from build123d import *

# Parameters (mm, degrees)
SKETCH_W        = 200
SKETCH_H        = 200
SKETCH_W_2      = 180
SKETCH_H_2      = 180
PAD_DEPTH       = 50
SKETCH001_W     = 40
SKETCH001_H     = 40
POCKET_DEPTH    = 2
SKETCH002_R     = 20
POCKET001_DEPTH = 8
SKETCH003_W     = 22
SKETCH003_H     = 12
POCKET002_DEPTH = 10
SKETCH004_R     = 5
POCKET003_DEPTH = 10
SKETCH005_W     = 15
SKETCH005_H     = 15
POCKET004_DEPTH = 2
SKETCH006_R     = 0.75
POCKET005_DEPTH = 10
POCKET006_DEPTH = 10
SKETCH008_W     = 10
SKETCH008_H     = 10
SKETCH008_R     = 1.8
PAD001_DEPTH    = 10
FILLET_R        = 1
SKETCH009_R     = 1.2
POCKET007_DEPTH = 5
SKETCH010_W     = 110
SKETCH010_H     = 40
POCKET008_DEPTH = 5
SKETCH011_W     = 110
SKETCH011_H     = 40
POCKET009_DEPTH = 5
SKETCH012_W     = 110
SKETCH012_H     = 40
POCKET010_DEPTH = 5


with BuildPart() as part:
    # Sketch → Pad (new body)
    with BuildSketch(Plane.XY):
        with Locations((100, 100)):
            Rectangle(SKETCH_W, SKETCH_H)
        with Locations((100, 100)):
            Rectangle(SKETCH_W_2, SKETCH_H_2, mode=Mode.SUBTRACT)
    extrude(amount=PAD_DEPTH)

    # Sketch001 (on Face1 of Pad) → Pocket (cut)
    with BuildSketch(Plane.XZ):
        with Locations((160, 25)):
            Rectangle(SKETCH001_W, SKETCH001_H)
    extrude(amount=-POCKET_DEPTH, mode=Mode.SUBTRACT)

    # Sketch002 (on Face15 of Pocket) → Pocket001 (cut)
    with BuildSketch(Plane.XZ.offset(-2)):
        with Locations((160, 25)):
            Circle(SKETCH002_R)
    extrude(amount=-POCKET001_DEPTH, mode=Mode.SUBTRACT)

    # Sketch003 (on Face1 of Pocket001) → Pocket002 (cut)
    with BuildSketch(Plane.XZ):
        with Locations((119, 11)):
            Rectangle(SKETCH003_W, SKETCH003_H)
    extrude(amount=-POCKET002_DEPTH, mode=Mode.SUBTRACT)

    # Sketch004 (on Face1 of Pocket002) → Pocket003 (cut)
    with BuildSketch(Plane.XZ):
        with Locations((93, 11)):
            Circle(SKETCH004_R)
    extrude(amount=-POCKET003_DEPTH, mode=Mode.SUBTRACT)

    # Sketch005 (on Face16 of Pocket003) → Pocket004 (cut)
    with BuildSketch(Plane(origin=(0, 10, 0), x_dir=(-1, 0, 0), z_dir=(0, 1, 0))):
        with Locations((-93, 11)):
            Rectangle(SKETCH005_W, SKETCH005_H)
    extrude(amount=-POCKET004_DEPTH, mode=Mode.SUBTRACT)

    # Sketch006 (on Face4 of Pocket004) → Pocket005 (cut)
    with BuildSketch(Plane.XY.offset(50)):
        with Locations((5, 5)):
            Circle(SKETCH006_R)
        with Locations((195, 5)):
            Circle(SKETCH006_R)
        with Locations((195, 195)):
            Circle(SKETCH006_R)
        with Locations((5, 195)):
            Circle(SKETCH006_R)
    extrude(amount=-POCKET005_DEPTH, mode=Mode.SUBTRACT)

    # Sketch007 (on Face15 of Pocket005) → Pocket006 (cut)
    with BuildSketch(Plane(origin=(0, 200, 0), x_dir=(-1, 0, 0), z_dir=(0, 1, 0))):
        with BuildLine():
            ThreePointArc((-38, 10), (-36.5, 8.5), (-35, 10))
            Line((-35, 10), (-35, 40))
            ThreePointArc((-35, 40), (-36.5, 41.5), (-38, 40))
            Line((-38, 10), (-38, 40))
        make_face()
        with BuildLine():
            ThreePointArc((-33, 10), (-31.5, 8.5), (-30, 10))
            Line((-30, 10), (-30, 40))
            ThreePointArc((-30, 40), (-31.5, 41.5), (-33, 40))
            Line((-33, 10), (-33, 40))
        make_face()
        with BuildLine():
            ThreePointArc((-28, 10), (-26.5, 8.5), (-25, 10))
            Line((-25, 10), (-25, 40))
            ThreePointArc((-25, 40), (-26.5, 41.5), (-28, 40))
            Line((-28, 10), (-28, 40))
        make_face()
        with BuildLine():
            ThreePointArc((-165, 10), (-163.5, 8.5), (-162, 10))
            Line((-162, 10), (-162, 40))
            ThreePointArc((-162, 40), (-163.5, 41.5), (-165, 40))
            Line((-165, 10), (-165, 40))
        make_face()
        with BuildLine():
            ThreePointArc((-170, 10), (-168.5, 8.5), (-167, 10))
            Line((-167, 10), (-167, 40))
            ThreePointArc((-167, 40), (-168.5, 41.5), (-170, 40))
            Line((-170, 10), (-170, 40))
        make_face()
        with BuildLine():
            ThreePointArc((-175, 10), (-173.5, 8.5), (-172, 10))
            Line((-172, 10), (-172, 40))
            ThreePointArc((-172, 40), (-173.5, 41.5), (-175, 40))
            Line((-175, 10), (-175, 40))
        make_face()
    extrude(amount=-POCKET006_DEPTH, mode=Mode.SUBTRACT)

    # Sketch008 (on Face3 of Pocket006) → Pad001 (join)
    with BuildSketch(Plane(origin=(0, 0, 0), x_dir=(1, 0, 0), z_dir=(0, 0, -1))):
        with Locations((185, -15)):
            Rectangle(SKETCH008_W, SKETCH008_H)
        with Locations((185, -15)):
            Circle(SKETCH008_R, mode=Mode.SUBTRACT)
        with Locations((185, -185)):
            Rectangle(SKETCH008_W, SKETCH008_H)
        with Locations((185, -185)):
            Circle(SKETCH008_R, mode=Mode.SUBTRACT)
        with Locations((15, -15)):
            Rectangle(SKETCH008_W, SKETCH008_H)
        with Locations((15, -15)):
            Circle(SKETCH008_R, mode=Mode.SUBTRACT)
        with Locations((15, -185)):
            Rectangle(SKETCH008_W, SKETCH008_H)
        with Locations((15, -185)):
            Circle(SKETCH008_R, mode=Mode.SUBTRACT)
    extrude(amount=-PAD001_DEPTH)

    # Fillet
    fillet_edges = [part.edges().sort_by_distance(p)[0] for p in [
        (180, 20, 5),
        (20, 20, 5),
        (180, 180, 5),
        (20, 180, 5),
    ]]
    fillet(fillet_edges, radius=FILLET_R)

    # Sketch009 (on Face8 of Fillet) → Pocket007 (cut)
    with BuildSketch(Plane(origin=(0, 10, 0), x_dir=(-1, 0, 0), z_dir=(0, 1, 0))):
        with Locations((-144, 9)):
            Circle(SKETCH009_R)
        with Locations((-176, 41)):
            Circle(SKETCH009_R)
        with Locations((-176, 9)):
            Circle(SKETCH009_R)
        with Locations((-144, 41)):
            Circle(SKETCH009_R)
    extrude(amount=-POCKET007_DEPTH, mode=Mode.SUBTRACT)

    # Sketch010 (on Face22 of Pocket007) → Pocket008 (cut)
    with BuildSketch(Plane.YZ.offset(200)):
        with Locations((100, 25)):
            Rectangle(SKETCH010_W, SKETCH010_H)
    extrude(amount=-POCKET008_DEPTH, mode=Mode.SUBTRACT)

    # Sketch011 (on Face20 of Pocket008) → Pocket009 (cut)
    with BuildSketch(Plane(origin=(0, 0, 0), x_dir=(0, -1, 0), z_dir=(-1, 0, 0))):
        with Locations((-100, 25)):
            Rectangle(SKETCH011_W, SKETCH011_H)
    extrude(amount=-POCKET009_DEPTH, mode=Mode.SUBTRACT)

    # Sketch012 (on Face21 of Pocket009) → Pocket010 (cut)
    with BuildSketch(Plane(origin=(0, 200, 0), x_dir=(-1, 0, 0), z_dir=(0, 1, 0))):
        with Locations((-100, 25)):
            Rectangle(SKETCH012_W, SKETCH012_H)
    extrude(amount=-POCKET010_DEPTH, mode=Mode.SUBTRACT)


solid = part.part
Work out the finished part from the listing and answer in its coordinate system (mm). A direction names the side the tool comes from. Coordinates: 2 decimals unless noted, no trailing zeros. Write each loop counter-clockwise with the first axis right and the second up, starting at its lowest first coordinate (ties: lowest second). Pieces come first, ordered by that corner, then holes. Notation, with made-up numbers: M 76,-20.75 L 130,-20.75 A17 ccw 130,-5.75 Z; hole C 60,16 d10. An arc over 180 degrees is marked long. Answer as CSV lines item,"result". Start each with the question number.
Item 1: Section D-D on z = 32 is taken. Give the number of separate pieces and of enclosed holes in the cut face, and give its area (3 significant figures).
Item 2: Determine the mould class of faces 4 (the face through (165, 195, 25)), 5 (the face through (176, 2, 9)), 6 (the face through (10, 99, 25)) for opening direction Y: released by +Y, released by -Y, zero draft, split by the parting line, or undercut.
Item 3: Section A-A on y = 70 is taken. Write down the section's boundary in (x, z).
Item 4: A tool of negligible diameter and unlimited length cuts with its end or side. For faces 1 (the face through (5, 101, 25)), 2 (the face through (14, 20, 5)), 3 (the face through (25, 195, 25)), from which of +Z, -Z, +X, -X, +Y, -Y can it reach the whole face along a straight path? Write none if from no direction.
Item 5: Consider L1, parallel to Y at x = 185, z = 4; L2, parallel to X at y = 62, z = 20.5. Determine where each line is inside the solid, lowest interval first.
Item 6: Flat-ended cylindrical pins translate along their axes: P1, Ø8, axis at y = 3.5, z = 13.5, coming from the -X side; P2, Ø25, axis at y = 74.5, z = 28.5, coming from the -X side; P3, Ø2, axis at y = 71.5, z = 18.5, coming from the +X side; P4, Ø6, axis at x = 168.5, z = 34, coming from the -Y side. Find the tip coordinate at first contact, or state that the pin passes through.
Item 7: Section B-B on x = 122.5 is taken. Write down the section's boundary in (y, z), and give its area (3 significant figures).
Item 8: Section C-C on x = 22.5 is taken. Write down the section's boundary in (y, z).
Checks:
1,separate pieces,"7"
1,enclosed holes,"0"
1,area,"5,390 mm²"
2,face 4,"zero draft"
2,face 5,"released by -Y"
2,face 6,"undercut"
3,outline,"M 0,0 L 10,0 L 10,50 L 0,50 L 0,45 L 5,45 L 5,5 L 0,5 Z; M 190,0 L 200,0 L 200,5 L 195,5 L 195,45 L 200,45 L 200,50 L 190,50 Z"
4,face 1,"-X"
4,face 2,"+Z, -Z"
4,face 3,"+Y"
5,L1,"y = 0 to 13.2, 16.8 to 20, 180 to 183.2, 186.8 to 200"
5,L2,"x = 5 to 10, 190 to 195"
6,P1,"stops at x = 0"
6,P2,"stops at x = 5"
6,P3,"stops at x = 195"
6,P4,"stops at y = 190"
7,outline,"M 0,0 L 10,0 L 10,5 L 0,5 Z; M 0,17 L 10,17 L 10,50 L 0,50 Z; M 190,0 L 200,0 L 200,5 L 195,5 L 195,45 L 200,45 L 200,50 L 190,50 Z"
7,area,"680 mm²"
8,outline,"M 0,0 L 10,0 L 10,50 L 0,50 Z; M 190,0 L 200,0 L 200,50 L 190,50 Z"
